Input: dimensioned drawing with shaded views. Units: mm. Origin: part minimum x, y, z. A direction names the side the tool comes from. Give positions to 0.01 mm unless a question says otherwise; leave off trailing zeros. Write each loop counter-clockwise with the first axis right and the second up, starting at its lowest first coordinate (ties: lowest second). Pieces come first, ordered by that corner, then holes.
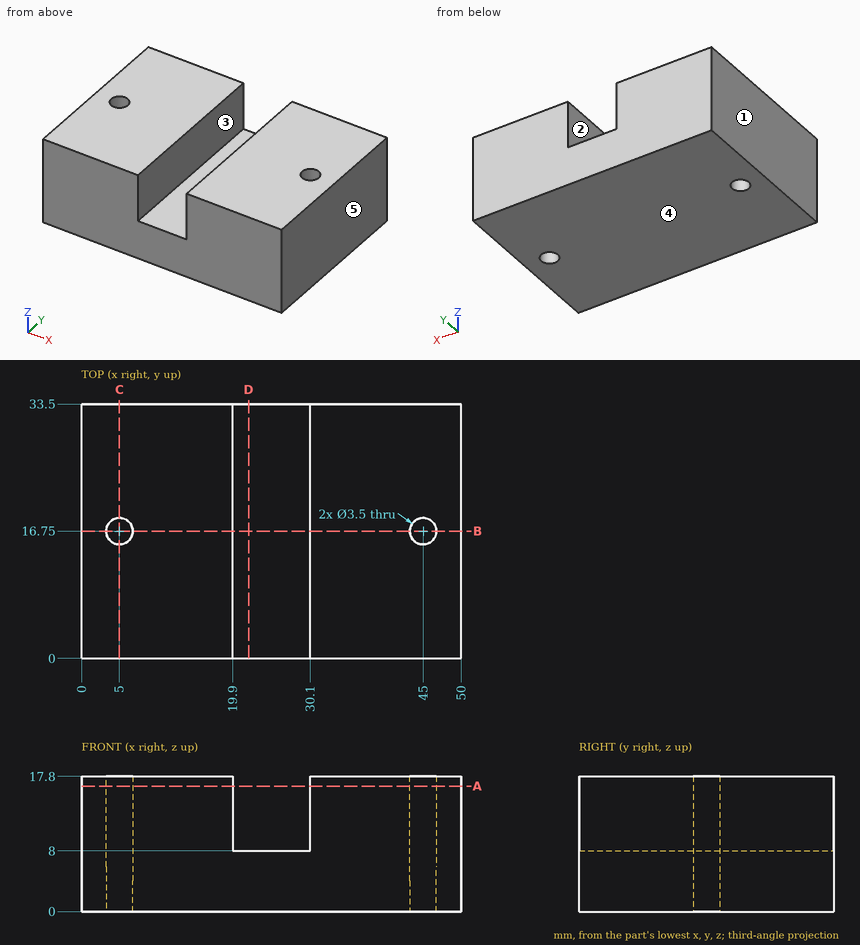
Item 1: Mould query, pull axis X, two halves, no side actions, for the marked faces 3, 4 and 5. Classes: +X half, -X half, draft (parallel to the pull), parting line (faces both ways), or undercut.
Item 2: Section C-C (x = 5). Return loops of the section in (y, z).
Item 3: Pin query (flat end, axial travel): pin 1 (8 mm diameter, centred on x = 25.5, y = 22, fed in from +Z). Return the tip coordinate at first contact, or that it passes through.
Item 4: Section A-A (z = 16.5). Return loops of the section in (x, y).
Item 5: Section B-B (y = 16.75). Return loops of the section in (x, z), and give its area (3 significant figures).
Item 6: Ray query, line 1 (X direction, y = 20, z = 16.5); line 2 (Y direction, x = 5, z = 9.75); line 3 (X direction, y = 16, z = 14.25). Return the intervals inside material, ascending.
Item 7: Set-up query: the marked faces 1 and 2. Return all of +Z, -Z, +X, -X, +Y, -Y with unobstructed straight access to the full face (end or side cutting, diameter ignored); none if empty.
Item 8: Section D-D (x = 22). Return loops of the section in (y, z).
Solved:
1. face 3: undercut
1. face 4: draft
1. face 5: +X half
2. outline: (0, 0) - (15, 0) - (15, 17.8) - (0, 17.8) - close; (18.5, 0) - (33.5, 0) - (33.5, 17.8) - (18.5, 17.8) - close
3. pin 1: stops at z = 8
4. outline: (0, 0) - (19.9, 0) - (19.9, 33.5) - (0, 33.5) - close; (30.1, 0) - (50, 0) - (50, 33.5) - (30.1, 33.5) - close; hole circle Ø3.5 at (5, 16.75); hole circle Ø3.5 at (45, 16.75)
5. outline: (0, 0) - (3.25, 0) - (3.25, 17.8) - (0, 17.8) - close; (6.75, 0) - (43.25, 0) - (43.25, 17.8) - (30.1, 17.8) - (30.1, 8) - (19.9, 8) - (19.9, 17.8) - (6.75, 17.8) - close; (46.75, 0) - (50, 0) - (50, 17.8) - (46.75, 17.8) - close
5. area: 665 mm2
6. line 1: x = 0 to 19.9, 30.1 to 50
6. line 2: y = 0 to 15, 18.5 to 33.5
6. line 3: x = 0 to 3.42, 6.58 to 19.9, 30.1 to 43.42, 46.58 to 50
7. face 1: +Z, -Z, -X, +Y, -Y
7. face 2: +Z, +Y, -Y
8. outline: (0, 0) - (33.5, 0) - (33.5, 8) - (0, 8) - close
